Could you check a few things on this drawing? It's one solid part, dimensions in mm from its lowest x, y, z. Round coordinates to 2 decimals unless told otherwise and drop trailing zeros. Loops run counter-clockwise (first coordinate to the right, second up) from the corner with the lowest first, then second, coordinate; pieces in that order, holes last. Notation, with made-up numbers: (7.25, -18.5) -> (54.25, -18.5) arc R12 ccw to (54.25, -14.5) -> close; hole circle Ø6 at (12, -25.75). An arc over 180 degrees is marked (long way). Use one line per item in the form item = value. Start each with the question number.
Item 1: If we section it at C-C (x = 53): Write out the boundary of the cut face in (y, z), then the cut area to 3 significant figures.
Item 2: If we section it at B-B (z = 8): Write out the boundary of the cut face in (x, y), then the cut area to 3 significant figures.
Item 3: I'm going to push flat-ended pins straight in: pin 1 Ø5.5 at (y, z) = (5.5, 43.5) entering from -X; pin 2 Ø1.5 at (x, z) = (12, 63.5) entering from +Y; pin 3 Ø1.5 at (x, y) = (74, 7) entering from +Z. Where does each tip first touch, or does it pass through?
Item 4: If we section it at D-D (z = 64): Write out the boundary of the cut face in (x, y).
Item 5: If I drill on L1, parallel to Z at x = 71, y = 3.75; L2, parallel to X at y = 6.5, z = 58.5; L3, parallel to Y at x = 46.5, z = 47, over which ranges is the centre line in solid material (lowest first)? Write a range as [from, to].
Item 6: Thinking about a two-plate mould opening in X: for the marked faces 1, 2 and 3, which applies, released by +X, released by -X, zero draft, split by the parting line, or undercut?
Item 7: If we section it at A-A (y = 4.5): Write out the boundary of the cut face in (x, z).
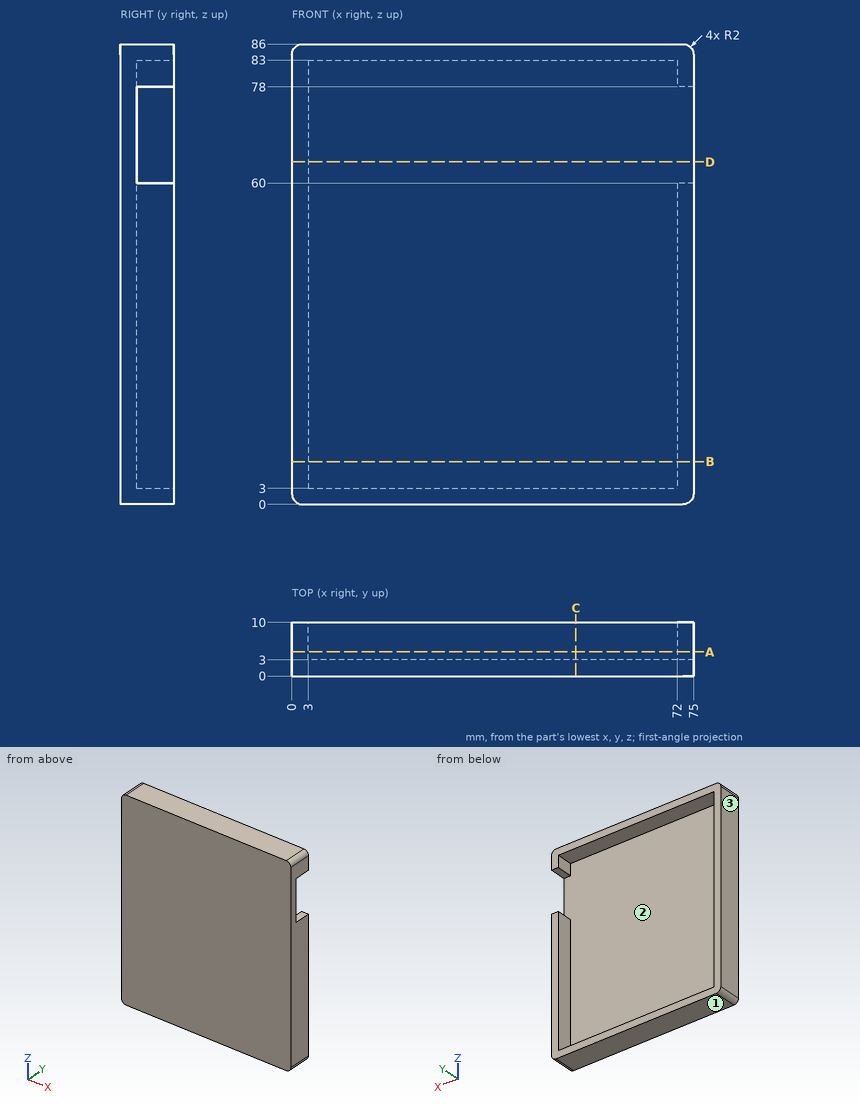
Values found:
q1.outline = (0, 0) -> (10, 0) -> (10, 3) -> (3, 3) -> (3, 83) -> (10, 83) -> (10, 86) -> (0, 86) -> close
q1.area = 300 mm2
q2.outline = (0, 0) -> (75, 0) -> (75, 10) -> (72, 10) -> (72, 3) -> (3, 3) -> (3, 10) -> (0, 10) -> close
q2.area = 267 mm2
q3.pin_1 = 0
q3.pin_2 = 3
q3.pin_3 = 85.98
q4.outline = (0, 0) -> (75, 0) -> (75, 3) -> (3, 3) -> (3, 10) -> (0, 10) -> close
q5.L1 = [0, 3], [83, 86]
q5.L2 = [0, 3], [72, 75]
q5.L3 = [0, 3]
q6.face_1 = zero draft
q6.face_2 = undercut
q6.face_3 = released by -X
q7.outline = (0, 2) arc R2 ccw to (2, 0) -> (73, 0) arc R2 ccw to (75, 2) -> (75, 60) -> (72, 60) -> (72, 3) -> (3, 3) -> (3, 83) -> (72, 83) -> (72, 78) -> (75, 78) -> (75, 84) arc R2 ccw to (73, 86) -> (2, 86) arc R2 ccw to (0, 84) -> close
